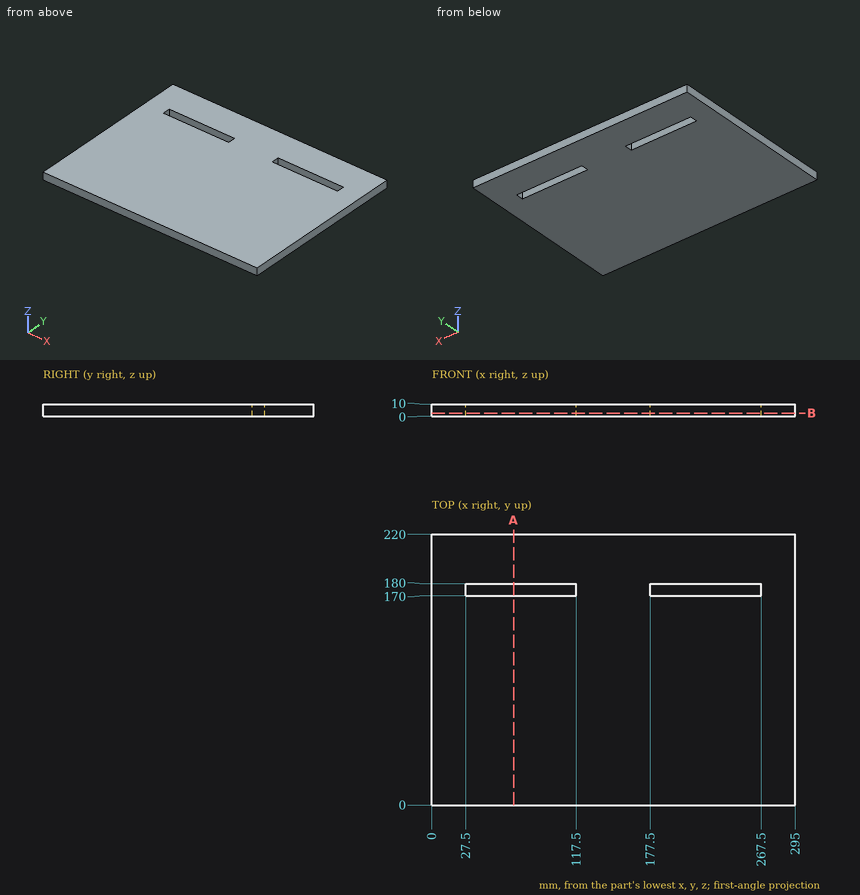
Could you check a few things on this drawing? It's one solid part, dimensions in mm from its lowest x, y, z. Give positions to 0.01 mm unless a question says otherwise; leave off trailing zeros. Write each loop counter-clockwise with the first axis right and the second up, starting at its lowest first coordinate (ties: lowest second). Pieces come first, ordered by that corner, then holes. Notation, with made-up numbers: (-8, -27.5) -> (28, -27.5) arc R33 cw to (28, 1.5) -> close; hole circle Ø9 at (27.5, -40). An arc over 180 degrees is marked (long way). Write item = value, one per line.
(1) Suppose I cut it at B-B on z = 2.5. Write out the boundary of the cut face in (x, y), then the cut area to 3 significant figures.
Worked out:
outline = (0, 0) -> (295, 0) -> (295, 220) -> (0, 220) -> close; hole (27.5, 170) -> (117.5, 170) -> (117.5, 180) -> (27.5, 180) -> close; hole (177.5, 170) -> (267.5, 170) -> (267.5, 180) -> (177.5, 180) -> close
area = 63,100 mm^2
(2) I need wall thicknesses on probe 1 along X at (y, z) = (175, 4); probe 2 along Y at (x, z) = (35.5, 9.5). Which ranges of each line are inside material? Lowest first, please. Write a range as from..to.
Worked out:
probe_1 = 0..27.5, 117.5..177.5, 267.5..295
probe_2 = 0..170, 180..220
(3) Suppose I cut it at A-A on x = 66.5. Write out the boundary of the cut face in (y, z).
Worked out:
outline = (0, 0) -> (170, 0) -> (170, 10) -> (0, 10) -> close; (180, 0) -> (220, 0) -> (220, 10) -> (180, 10) -> close
(4) I'm going to push a flat-ended pin straight in: P1, Ø3, axis at x = 227.5, z = 4.5, coming from the -Y side. Where does the tip first touch, or does it pass through?
Worked out:
P1 = 0
